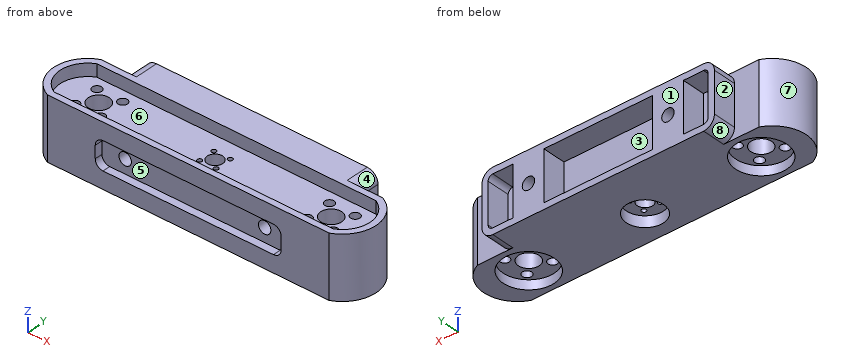
Autodesk Inventor part; units mm, degrees
ref_plane "YZ Plane" through (0, 0, 0) normal (1, 0, 0) x (0, 1, 0)
ref_plane "XZ Plane" through (0, 0, 0) normal (0, 1, 0) x (-1, 0, 0)
ref_plane "XY Plane" through (0, 0, 0) normal (0, 0, 1) x (1, 0, 0)
sketch "Sketch1" plane through (0, 0, 0) normal (0, 0, 1) x (1, 0, 0)
  circle A0 centre (75, 0) radius 15.85 construction
  circle A1 centre (66.6915, 8.3085) radius 3
  circle A2 centre (83.3085, -8.3085) radius 3
  circle A3 centre (66.6915, -8.3085) radius 3
  circle A4 centre (83.3085, 8.3085) radius 3
  circle A5 centre (75, 0) radius 6.75
  circle A6 centre (-75, 0) radius 15.85 construction
  circle A7 centre (-83.3085, 8.3085) radius 3
  circle A8 centre (-66.6915, -8.3085) radius 3
  circle A9 centre (-83.3085, -8.3085) radius 3
  circle A10 centre (-66.6915, 8.3085) radius 3
  circle A11 centre (-75, 0) radius 6.75
  circle A12 centre (5.3033, -5.3033) radius 1.5
  circle A13 centre (-5.3033, 5.3033) radius 1.5
  circle A14 centre (-5.3033, -5.3033) radius 1.5
  circle A15 centre (5.3033, 5.3033) radius 1.5
  circle A16 centre (0, 0) radius 10.75 construction
  circle A17 centre (0, 0) radius 5
  line L0 (100, -16) -> (-100, -16) construction
  line L1 (-100, -16) -> (-100, 16) construction
  line L2 (-100, 16) -> (100, 16) construction
  line L3 (100, 16) -> (100, -16) construction
  line L4 (100, -16) -> (-100, 16) construction
  line L5 (-100, -16) -> (100, 16) construction
  line L6 (0, 16) -> (-90, 16)
  line L7 (0, -16) -> (-90, -16)
  arc A18 (-90, 16) -> (-90, -16) centre (-82.2, 0) ccw
  line L8 (0, 16) -> (90, 16)
  line L9 (0, -16) -> (90, -16)
  arc A19 (90, -16) -> (90, 16) centre (82.2, 0) ccw
  point P0 (0, 0)
  point P1 (75, 0)
  point P2 (-75, 0)
  dimension "d4" = 10
  dimension "d5" = 75
  dimension "d6" = 75
  dimension "d7" = 200
  dimension "d8" = 32
  dimension "d9" = 90
  dimension "d10" = 90
  dimension "d11" = 90
  dimension "d12" = 90
extrude "Extrusion1" add sketch "Sketch1" along normal blind 30
sketch "Sketch2" plane through (0, 0, 0) normal (0, 0, -1) x (-1, 0, 0)
  circle A0 centre (75, 0) radius 6.75 construction
  circle A1 centre (-75, 0) radius 6.75 construction
  circle A2 centre (0, 0) radius 5 construction
  circle A3 centre (66.6915, 8.3085) radius 3 construction
  circle A4 centre (83.3085, -8.3085) radius 3 construction
  circle A5 centre (66.6915, -8.3085) radius 3 construction
  circle A6 centre (83.3085, 8.3085) radius 3 construction
  circle A7 centre (-83.3085, 8.3085) radius 3 construction
  circle A8 centre (-66.6915, -8.3085) radius 3 construction
  circle A9 centre (-83.3085, -8.3085) radius 3 construction
  circle A10 centre (-66.6915, 8.3085) radius 3 construction
  circle A11 centre (-5.3033, 5.3033) radius 1.5 construction
  circle A12 centre (5.3033, -5.3033) radius 1.5 construction
  circle A13 centre (5.3033, 5.3033) radius 1.5 construction
  circle A14 centre (-5.3033, -5.3033) radius 1.5 construction
  line L0 (-90, 16) -> (90, 16)
  arc A15 (-90, 16) -> (-90, -16) centre (-82.2, 0) ccw
  line L1 (90, -16) -> (-90, -16)
  arc A16 (90, -16) -> (90, 16) centre (82.2, 0) ccw
  line L2 (90.8741, 20) -> (-90.8741, 20)
  arc A17 (-90.8741, 20) -> (-90.8741, -20) centre (-82.2, 0) ccw
  line L3 (-90.8741, -20) -> (90.8741, -20)
  arc A18 (90.8741, -20) -> (90.8741, 20) centre (82.2, 0) ccw
  dimension "d15" = 4
extrude "Extrusion2" add sketch "Sketch2" against normal blind 30
sketch "Sketch3" plane through (0, 0, 0) normal (0, 0, -1) x (-1, 0, 0)
  line L0 (90.8741, 20) -> (-90.8741, 20) construction
  arc A0 (-90.8741, 20) -> (-90.8741, -20) centre (-82.2, 0) ccw construction
  line L1 (-90.8741, -20) -> (90.8741, -20) construction
  arc A1 (90.8741, -20) -> (90.8741, 20) centre (82.2, 0) ccw construction
  circle A2 centre (75, 0) radius 6.75 construction
  circle A3 centre (-75, 0) radius 6.75 construction
  circle A4 centre (0, 0) radius 5 construction
  circle A5 centre (66.6915, 8.3085) radius 3 construction
  circle A6 centre (83.3085, -8.3085) radius 3 construction
  circle A7 centre (66.6915, -8.3085) radius 3 construction
  circle A8 centre (83.3085, 8.3085) radius 3 construction
  circle A9 centre (-83.3085, 8.3085) radius 3 construction
  circle A10 centre (-66.6915, -8.3085) radius 3 construction
  circle A11 centre (-83.3085, -8.3085) radius 3 construction
  circle A12 centre (-66.6915, 8.3085) radius 3 construction
  circle A13 centre (-5.3033, 5.3033) radius 1.5 construction
  circle A14 centre (5.3033, -5.3033) radius 1.5 construction
  circle A15 centre (5.3033, 5.3033) radius 1.5 construction
  circle A16 centre (-5.3033, -5.3033) radius 1.5 construction
  circle A17 centre (0, 0) radius 12
  circle A18 centre (-75, 0) radius 16.5
  circle A19 centre (75, 0) radius 16.5
  dimension "d18" = 24
  dimension "d19" = 33
  dimension "d20" = 33
extrude "Extrusion3" cut sketch "Sketch3" against normal blind 5
sketch "Sketch4" plane through (0, 0, 30) normal (0, 0, 1) x (1, 0, 0)
  line L0 (90.8741, 20) -> (-90.8741, 20) construction
  arc A0 (-90.8741, 20) -> (-90.8741, -20) centre (-82.2, 0) ccw construction
  line L1 (-90.8741, -20) -> (90.8741, -20) construction
  arc A1 (90.8741, -20) -> (90.8741, 20) centre (82.2, 0) ccw construction
  circle A2 centre (-75, 0) radius 6.75 construction
  circle A3 centre (75, 0) radius 6.75 construction
  circle A4 centre (0, 0) radius 5 construction
  circle A5 centre (-66.6915, 8.3085) radius 3 construction
  circle A6 centre (-83.3085, -8.3085) radius 3 construction
  circle A7 centre (-66.6915, -8.3085) radius 3 construction
  circle A8 centre (-83.3085, 8.3085) radius 3 construction
  circle A9 centre (83.3085, 8.3085) radius 3 construction
  circle A10 centre (66.6915, -8.3085) radius 3 construction
  circle A11 centre (83.3085, -8.3085) radius 3 construction
  circle A12 centre (66.6915, 8.3085) radius 3 construction
  circle A13 centre (5.3033, 5.3033) radius 1.5 construction
  circle A14 centre (-5.3033, -5.3033) radius 1.5 construction
  circle A15 centre (-5.3033, 5.3033) radius 1.5 construction
  circle A16 centre (5.3033, -5.3033) radius 1.5 construction
  line L2 (90, -16) -> (-90, -16)
  arc A17 (-90, 16) -> (-90, -16) centre (-82.2, 0) ccw
  line L3 (-90, 16) -> (90, 16)
  arc A18 (90, -16) -> (90, 16) centre (82.2, 0) ccw
  dimension "d23" = 4
extrude "Extrusion4" cut sketch "Sketch4" against normal blind 5
sketch "Sketch5" plane through (0, 0, 5) normal (0, 0, -1) x (-1, 0, 0)
  circle A0 centre (0, 0) radius 5
  circle A1 centre (-5.3033, 5.3033) radius 1.5
  circle A2 centre (5.3033, -5.3033) radius 1.5
  circle A3 centre (5.3033, 5.3033) radius 1.5
  circle A4 centre (-5.3033, -5.3033) radius 1.5
  circle A5 centre (0, 0) radius 12
extrude "Extrusion5" cut sketch "Sketch5" against normal blind 2
sketch "Sketch6" plane through (-75, 0, 5) normal (0, 0, -1) x (-1, 0, 0)
  circle A0 centre (0, 0) radius 6.75
  circle A1 centre (-8.3085, 8.3085) radius 3
  circle A2 centre (8.3085, -8.3085) radius 3
  circle A3 centre (-8.3085, -8.3085) radius 3
  circle A4 centre (8.3085, 8.3085) radius 3
  circle A5 centre (0, 0) radius 16.5
  circle A6 centre (-150, 0) radius 6.75
  circle A7 centre (-158.3085, 8.3085) radius 3
  circle A8 centre (-141.6915, -8.3085) radius 3
  circle A9 centre (-158.3085, -8.3085) radius 3
  circle A10 centre (-141.6915, 8.3085) radius 3
  circle A11 centre (-150, 0) radius 16.5
  point P0 (-75, 0)
extrude "Extrusion6" cut sketch "Sketch6" against normal blind 1
sketch "Sketch7" plane through (0, 0, 30) normal (0, 0, 1) x (1, 0, 0)
  arc A0 (90, -16) -> (90, 16) centre (82.2, 0) ccw
  line L0 (90, -16) -> (-90, -16)
  arc A1 (-90, 16) -> (-90, -16) centre (-82.2, 0) ccw
  line L1 (-90, 16) -> (90, 16)
  line L2 (90.8741, 20) -> (-90.8741, 20)
  arc A2 (-90.8741, 20) -> (-90.8741, -20) centre (-82.2, 0) ccw
  line L3 (-90.8741, -20) -> (90.8741, -20)
  arc A3 (90.8741, -20) -> (90.8741, 20) centre (82.2, 0) ccw
  point P0 (0, 0)
extrude "Extrusion7" add sketch "Sketch7" along normal blind 10
sketch "Sketch8" plane through (0, 0, 25) normal (0, 0, 1) x (1, 0, 0)
  circle A0 centre (-75, 0) radius 6.75
  circle A1 centre (75, 0) radius 6.75
  circle A2 centre (0, 0) radius 5
  circle A3 centre (-66.6915, 8.3085) radius 3
  circle A4 centre (-83.3085, -8.3085) radius 3
  circle A5 centre (-66.6915, -8.3085) radius 3
  circle A6 centre (-83.3085, 8.3085) radius 3
  circle A7 centre (83.3085, 8.3085) radius 3
  circle A8 centre (66.6915, -8.3085) radius 3
  circle A9 centre (83.3085, -8.3085) radius 3
  circle A10 centre (66.6915, 8.3085) radius 3
  circle A11 centre (5.3033, 5.3033) radius 1.5
  circle A12 centre (-5.3033, -5.3033) radius 1.5
  circle A13 centre (-5.3033, 5.3033) radius 1.5
  circle A14 centre (5.3033, -5.3033) radius 1.5
  line L0 (90, -16) -> (-90, -16)
  arc A15 (90, -16) -> (90, 16) centre (82.2, 0) ccw
  line L1 (-90, 16) -> (90, 16)
  arc A16 (-90, 16) -> (-90, -16) centre (-82.2, 0) ccw
extrude "Extrusion8" add sketch "Sketch8" along normal blind 7
sketch "Sketch10" plane through (-90.8741, 20, 0) normal (0, 1, 0) x (1, 0, 0)
  circle A0 centre (135.8741, -20) radius 4
  circle A1 centre (150.8741, -20) radius 4 construction
  circle A2 centre (30.8741, -20) radius 4 construction
  circle A3 centre (45.8741, -20) radius 4
  arc A4 (15.8741, -33) -> (22.8741, -40) centre (22.8741, -33) ccw
  line L0 (22.8741, -40) -> (158.8741, -40)
  arc A5 (158.8741, -40) -> (165.8741, -33) centre (158.8741, -33) ccw
  line L1 (165.8741, -33) -> (165.8741, -7)
  arc A6 (165.8741, -7) -> (158.8741, 0) centre (158.8741, -7) ccw
  line L2 (158.8741, 0) -> (22.8741, 0)
  arc A7 (22.8741, 0) -> (15.8741, -7) centre (22.8741, -7) ccw
  line L3 (15.8741, -7) -> (15.8741, -33)
  line L4 (0, 0) -> (181.7482, 0) construction
  line L5 (0, 0) -> (0, -40) construction
  line L6 (181.7482, -40) -> (0, -40) construction
  line L7 (181.7482, 0) -> (181.7482, -40) construction
  line L8 (180.8741, -40) -> (0.8741, -40) construction
  line L9 (90.8741, -40) -> (90.8741, 0) construction
  line L10 (90.8741, 0) -> (90.8741, -40) construction
  line L11 (161.8741, -7) -> (161.8741, -33)
  arc A8 (158.8741, -36) -> (161.8741, -33) centre (158.8741, -33) ccw
  arc A9 (19.8741, -33) -> (22.8741, -36) centre (22.8741, -33) ccw
  line L12 (19.8741, -33) -> (19.8741, -7)
  arc A10 (22.8741, -4) -> (19.8741, -7) centre (22.8741, -7) ccw
  arc A11 (161.8741, -7) -> (158.8741, -4) centre (158.8741, -7) ccw
  line L13 (135.8741, -20) -> (135.8741, -36) construction
  line L14 (135.8741, -20) -> (135.8741, -4) construction
  line L15 (45.8741, -20) -> (45.8741, -36) construction
  line L16 (45.8741, -20) -> (45.8741, -4) construction
  line L17 (145.8741, -4) -> (145.8741, -36)
  line L18 (125.8741, -36) -> (125.8741, -4)
  line L19 (125.8741, -4) -> (145.8741, -36) construction
  line L20 (145.8741, -4) -> (125.8741, -36) construction
  line L21 (55.8741, -4) -> (55.8741, -36)
  line L22 (35.8741, -36) -> (35.8741, -4)
  line L23 (35.8741, -4) -> (55.8741, -36) construction
  line L24 (55.8741, -4) -> (35.8741, -36) construction
  line L25 (158.8741, -36) -> (145.8741, -36)
  line L26 (125.8741, -36) -> (55.8741, -36)
  line L27 (145.8741, -4) -> (158.8741, -4)
  line L28 (149.3741, 0) -> (149.3741, -6)
  line L29 (125.8741, -4) -> (55.8741, -4)
  line L30 (35.8741, -4) -> (22.8741, -4)
  line L31 (35.8741, -36) -> (22.8741, -36)
  line L32 (35.8741, -4) -> (35.8741, -36)
  line L33 (35.8741, -36) -> (22.8741, -36)
  arc A12 (19.8741, -33) -> (22.8741, -36) centre (22.8741, -33) ccw
  line L34 (19.8741, -33) -> (19.8741, -7)
  arc A13 (22.8741, -4) -> (19.8741, -7) centre (22.8741, -7) ccw
  line L35 (22.8741, -4) -> (35.8741, -4)
  point P0 (20, -7)
  dimension "d47" = 4
  dimension "d48" = 20
  dimension "d49" = 20
extrude "Extrusion11" add sketch "Sketch10" along normal blind 15
sketch "Sketch11" plane through (-45, 20, 20) normal (0, 1, 0) x (1, 0, 0)
  circle A0 centre (0, 0) radius 4
  circle A1 centre (90, 0) radius 4
  point P0 (45, 20)
extrude "Extrusion12" cut sketch "Sketch11" against normal blind 85
sketch "Sketch12" plane through (-90.8741, -20, 0) normal (0, -1, 0) x (1, 0, 0)
  circle A0 centre (45.8741, 20) radius 4 construction
  circle A1 centre (135.8741, 20) radius 4 construction
  line L0 (181.7482, 0) -> (0, 0) construction
  line L1 (181.7482, 0) -> (181.7482, 40) construction
  line L2 (0, 40) -> (181.7482, 40) construction
  line L3 (0, 0) -> (0, 40) construction
  line L4 (90.8741, 0) -> (90.8741, 40) construction
  line L5 (0, 0) -> (0, 40) construction
  line L6 (0, 20) -> (181.7482, 20) construction
  line L7 (145.8741, 11) -> (35.8741, 11)
  line L8 (30.8741, 16) -> (30.8741, 24)
  line L9 (35.8741, 29) -> (145.8741, 29)
  line L10 (150.8741, 24) -> (150.8741, 16)
  line L11 (150.8741, 11) -> (30.8741, 29) construction
  line L12 (30.8741, 11) -> (150.8741, 29) construction
  arc A2 (35.8741, 29) -> (30.8741, 24) centre (35.8741, 24) ccw
  arc A3 (30.8741, 16) -> (35.8741, 11) centre (35.8741, 16) ccw
  arc A4 (150.8741, 24) -> (145.8741, 29) centre (145.8741, 24) ccw
  arc A5 (145.8741, 11) -> (150.8741, 16) centre (145.8741, 16) ccw
  point P0 (90.8741, 20)
  dimension "d54" = 120
  dimension "d55" = 18
  dimension "d56" = 5
extrude "Extrusion13" cut sketch "Sketch12" against normal blind 5
properties part number "Corredera" material "PC/ABS Plastic"
Input: part model. Units: mm. Frame: model coordinates. Face numbers are marked on the shaded views. A direction names the side the tool comes from. Give positions to 0.01 mm unless a question says otherwise; leave off trailing zeros. Loops run counter-clockwise (first coordinate to the right, second up) from the corner with the lowest first, then second, coordinate; pieces in that order, holes last. Notation, with made-up numbers: M -2.5,28.5 L 28.5,28.5 A15 cw 28.5,57.5 Z; hole C 46.25,34.5 d8. An arc over 180 degrees is marked long. Use one line per item in the form item = value.
1. Section query C-C, the plane z = 20. Count the separate pieces of the cut face and the enclosed holes in it, and give its area (3 significant figures).
Numbers:
separate_pieces = 3
enclosed_holes = 15
area = 6,730 mm²
2. Reachability of the marked faces 1, 2, 3 and 4 from +Z, -Z, +X, -X, +Y, -Y: full face, straight path, thin tool, end or side. Return the list, or none.
Numbers:
face_1 = +Z, -Z, +X, -X, +Y
face_2 = +Z, -Z, -X, +Y
face_3 = +Y
face_4 = +Z, +X, +Y
3. First-contact query: pin 1 (4 mm diameter, centred on y = 26, z = 18, fed in from -X); pin 2 (5.5 mm diameter, centred on y = -17, z = 20.5, fed in from +X); pin 3 (4 mm diameter, centred on x = -34, z = 21, fed in from -Y). Flat tips, straight axial feed; report the tip coordinate or a pass-through.
Numbers:
pin_1 = -75
pin_2 = 98.7
pin_3 = -15
4. Pull-direction query (Z, two-part tool) for the marked faces 5, 6, 7 and 8; classes: released by +Z, released by -Z, zero draft, split by the parting line, or undercut.
Numbers:
face_5 = undercut
face_6 = released by +Z
face_7 = zero draft
face_8 = released by -Z
5. Section query A-A, the plane y = 23.5. Return the cut outline in (x, z).
Numbers:
outline = M -75,7 A7 ccw -68,0 L 68,0 A7 ccw 75,7 L 75,33 A7 ccw 68,40 L -68,40 A7 ccw -75,33 Z; hole M -71,7 A3 ccw -68,4 L -55,4 L -55,36 L -68,36 A3 ccw -71,33 Z; hole C -45,20 d8; hole M -35,4 L 35,4 L 35,36 L -35,36 Z; hole C 45,20 d8; hole M 55,4 L 68,4 A3 ccw 71,7 L 71,33 A3 ccw 68,36 L 55,36 Z
6. Section query D-D, the plane x = -18. Return the cut outline in (y, z), and give its area (3 significant figures).
Numbers:
outline = M -20,0 L 35,0 L 35,4 L 20,4 L 20,36 L 35,36 L 35,40 L 16,40 L 16,32 L -16,32 L -16,40 L -20,40 L -20,29 L -15,29 L -15,11 L -20,11 Z
area = 1,370 mm²
7. Line query: L1, parallel to X at y = 25, z = 30; L2, parallel to Z at x = 68, y = 31.5; L3, parallel to X at y = -0.5, z = 25. Output: solid intervals per line, ascending.
Numbers:
L1 = -75 to -71, -55 to -35, 35 to 55, 71 to 75
L2 = 0 to 4, 36 to 40
L3 = -103.99 to -81.73, -68.27 to -4.97, 4.97 to 68.27, 81.73 to 103.99
8. Section query B-B, the plane x = 45. Return the cut outline in (y, z).
Numbers:
outline = M -20,0 L 35,0 L 35,16 L -15,16 L -15,11 L -20,11 Z; M -20,29 L -15,29 L -15,24 L 35,24 L 35,40 L 16,40 L 16,32 L -16,32 L -16,40 L -20,40 Z
